from build123d import *

# Parameters (mm, degrees)
BOSS_EXTRUDE2_DEPTH = 3.175


with BuildPart() as part:
    # Sketch1 → Boss-Extrude2 (new body)
    # profile 1 of 7: a face of its own
    with BuildSketch(Plane(origin=(0, 0, 0), x_dir=(1, 0, 0), z_dir=(0, 1, 0))):
        with BuildLine():
            ThreePointArc((28.575, -5.499261314), (31.75, 0), (28.575, 5.499261314))
            ThreePointArc((28.575, 5.499261314), (5.55625, 9.6237073), (-9.525, 27.49630657))
            ThreePointArc((-9.525, 27.49630657), (-15.875, 27.49630657), (-19.05, 21.997045256))
            ThreePointArc((-19.05, 21.997045256), (-11.443597622, 4.764679711), (-14.037901317, -13.892259152))
            Line((-14.037901317, -13.892259152), (-12.274630657, -14.910283942))
            ThreePointArc((-12.274630657, -14.910283942), (-11.1125, -13.748153285), (-9.525, -13.322783942))
            Line((-9.525, -13.322783942), (-9.525, 13.322783942))
            ThreePointArc((-9.525, 13.322783942), (-11.77006403, 18.742847972), (-6.35, 16.497783942))
            ThreePointArc((-6.35, 16.497783942), (-6.458185502, 15.676033474), (-6.775369343, 14.910283942))
            Line((-6.775369343, 14.910283942), (16.300369343, 1.5875))
            ThreePointArc((16.300369343, 1.5875), (19.871750468, 3.066814498), (22.225, 0))
            ThreePointArc((22.225, 0), (19.871750468, -3.066814498), (16.300369343, -1.5875))
            Line((16.300369343, -1.5875), (-6.775369343, -14.910283942))
            ThreePointArc((-6.775369343, -14.910283942), (-6.458185502, -15.676033474), (-6.35, -16.497783942))
            ThreePointArc((-6.35, -16.497783942), (-6.458185502, -17.31953441), (-6.775369343, -18.085283942))
            Line((-6.775369343, -18.085283942), (-5.012098683, -19.103308732))
            ThreePointArc((-5.012098683, -19.103308732), (9.848132482, -7.528106395), (28.575, -5.499261314))
        make_face()
    # profile 2 of 7: a face of its own
    with BuildSketch(Plane(origin=(0, 0, 0), x_dir=(1, 0, 0), z_dir=(0, 1, 0))):
        with BuildLine():
            ThreePointArc((-9.525, -27.49630657), (-7.560164077, -23.143006881), (-5.012098683, -19.103308732))
            Line((-5.012098683, -19.103308732), (-6.775369343, -18.085283942))
            ThreePointArc((-6.775369343, -18.085283942), (-11.1125, -19.247414599), (-12.274630657, -14.910283942))
            Line((-12.274630657, -14.910283942), (-14.037901317, -13.892259152))
            ThreePointArc((-14.037901317, -13.892259152), (-16.262349841, -18.118797588), (-19.05, -21.997045256))
            ThreePointArc((-19.05, -21.997045256), (-15.875, -27.49630657), (-9.525, -27.49630657))
        make_face()
    # profile 3 of 7: a face of its own
    with BuildSketch(Plane(origin=(0, 0, 0), x_dir=(1, 0, 0), z_dir=(0, 1, 0))):
        with BuildLine():
            Line((-9.525, 13.322783942), (-9.525, -13.322783942))
            ThreePointArc((-9.525, -13.322783942), (-7.9375, -13.748153285), (-6.775369343, -14.910283942))
            Line((-6.775369343, -14.910283942), (16.300369343, -1.5875))
            ThreePointArc((16.300369343, -1.5875), (15.875, 0), (16.300369343, 1.5875))
            Line((16.300369343, 1.5875), (-6.775369343, 14.910283942))
            ThreePointArc((-6.775369343, 14.910283942), (-7.9375, 13.748153285), (-9.525, 13.322783942))
        make_face()
        with BuildLine():
            Line((-8.065819658, -1.523195628), (-8.065819658, 1.523195628))
            Line((-8.065819658, 1.523195628), (-6.298644043, 1.523195628))
            ThreePointArc((-6.298644043, 1.523195628), (-5.996260328, 2.457214638), (-5.55625, 3.334835474))
            Line((-5.55625, 3.334835474), (-5.55625, 8.0362073))
            ThreePointArc((-5.55625, 8.0362073), (-6.678782015, 10.746239315), (-3.96875, 9.6237073))
            ThreePointArc((-3.96875, 9.6237073), (-4.022842751, 9.212832065), (-4.181434671, 8.8299573))
            Line((-4.181434671, 8.8299573), (-0.109927238, 6.479271387))
            ThreePointArc((-0.109927238, 6.479271387), (3.240101916, 5.61202114), (5.666177238, 3.144435913))
            Line((5.666177238, 3.144435913), (9.737684671, 0.79375))
            ThreePointArc((9.737684671, 0.79375), (11.523375234, 1.533407249), (12.7, 0))
            ThreePointArc((12.7, 0), (11.523375234, -1.533407249), (9.737684671, -0.79375))
            Line((9.737684671, -0.79375), (5.666177238, -3.144435913))
            ThreePointArc((5.666177238, -3.144435913), (3.240101916, -5.61202114), (-0.109927238, -6.479271387))
            Line((-0.109927238, -6.479271387), (-4.181434671, -8.8299573))
            ThreePointArc((-4.181434671, -8.8299573), (-4.022842751, -9.212832065), (-3.96875, -9.6237073))
            ThreePointArc((-3.96875, -9.6237073), (-6.678782015, -10.746239315), (-5.55625, -8.0362073))
            Line((-5.55625, -8.0362073), (-5.55625, -3.334835474))
            ThreePointArc((-5.55625, -3.334835474), (-5.996260328, -2.457214638), (-6.298644043, -1.523195628))
            Line((-6.298644043, -1.523195628), (-8.065819658, -1.523195628))
        make_face(mode=Mode.SUBTRACT)
    # profile 4 of 7: a face of its own
    with BuildSketch(Plane(origin=(0, 0, 0), x_dir=(1, 0, 0), z_dir=(0, 1, 0))):
        with BuildLine():
            Line((-5.55625, 8.0362073), (-5.55625, 3.334835474))
            ThreePointArc((-5.55625, 3.334835474), (-3.240101916, 5.61202114), (-0.109927238, 6.479271387))
            Line((-0.109927238, 6.479271387), (-4.181434671, 8.8299573))
            ThreePointArc((-4.181434671, 8.8299573), (-4.7625, 8.248891971), (-5.55625, 8.0362073))
        make_face()
    # profile 5 of 7: a face of its own
    with BuildSketch(Plane(origin=(0, 0, 0), x_dir=(1, 0, 0), z_dir=(0, 1, 0))):
        with BuildLine():
            ThreePointArc((-0.109927238, -6.479271387), (-3.240101916, -5.61202114), (-5.55625, -3.334835474))
            Line((-5.55625, -3.334835474), (-5.55625, -8.0362073))
            ThreePointArc((-5.55625, -8.0362073), (-4.7625, -8.248891971), (-4.181434671, -8.8299573))
            Line((-4.181434671, -8.8299573), (-0.109927238, -6.479271387))
        make_face()
    # profile 6 of 7: a face of its own
    with BuildSketch(Plane(origin=(0, 0, 0), x_dir=(1, 0, 0), z_dir=(0, 1, 0))):
        with BuildLine():
            ThreePointArc((5.666177238, 3.144435913), (6.037080593, 2.355143226), (6.298644043, 1.523195628))
            Line((6.298644043, 1.523195628), (8.065819658, 1.523195628))
            Line((8.065819658, 1.523195628), (8.065819658, -1.523195628))
            Line((8.065819658, -1.523195628), (6.298644043, -1.523195628))
            ThreePointArc((6.298644043, -1.523195628), (6.037080593, -2.355143226), (5.666177238, -3.144435913))
            Line((5.666177238, -3.144435913), (9.737684671, -0.79375))
            ThreePointArc((9.737684671, -0.79375), (9.525, 0), (9.737684671, 0.79375))
            Line((9.737684671, 0.79375), (5.666177238, 3.144435913))
        make_face()
    # profile 7 of 7: a face of its own
    with BuildSketch(Plane(origin=(0, 0, 0), x_dir=(1, 0, 0), z_dir=(0, 1, 0))):
        with BuildLine():
            Line((-6.298644043, 1.523195628), (-8.065819658, 1.523195628))
            Line((-8.065819658, 1.523195628), (-8.065819658, -1.523195628))
            Line((-8.065819658, -1.523195628), (-6.298644043, -1.523195628))
            ThreePointArc((-6.298644043, -1.523195628), (-6.480203832, 0), (-6.298644043, 1.523195628))
        make_face()
    extrude(amount=BOSS_EXTRUDE2_DEPTH)


solid = part.part
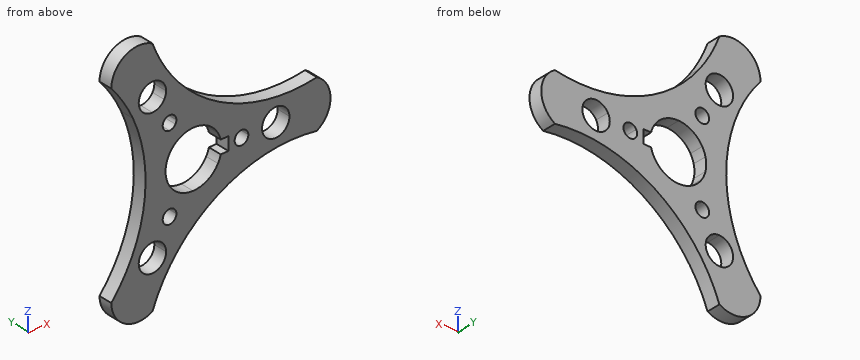
Could you check a few things on this model? Use its own coordinates, in mm. Give positions to 0.01 mm unless a question says otherwise; leave off trailing zeros. Order: outer loops, then holes, each group sorted by start corner. A loop starts at its lowest first (then second) coordinate and runs counter-clockwise, first axis right, second up. Notation, with made-up numbers: (-32.75, 10) - (-19.75, 10) arc R30 ccw to (-19.75, 45) - close; hole circle Ø8 at (-0.5, 1). An arc over 180 degrees is marked (long way). Return JSON: item names as keys, results as strings. Group by question number.
Q1. Will these pins go through, and if not, where does the flat tip stop? pin 1 Ø0.5 at (x, y) = (7.5, 2.5) entering from +Z; pin 2 Ø0.9 at (y, z) = (2, 0.5) entering from -X; pin 3 Ø1.4 at (x, y) = (7, 1.5) entering from -Z.
Q2. Suppose I cut it at B-B, the plane z = -10.5. Please give me the cut outline in (x, y) (3 decimals), and give its area (3 significant figures).
Q3. Suppose I cut it at C-C, the plane x = 2. Please give me the cut outline in (y, z) (3 decimals).
Q4. Please list where these lines run through material, in increasing order: line 1 along Z through (x, y) = (-9, 1.9); line 2 along Z through (x, y) = (-7, 0.55); line 3 along Z through (x, y) = (-6, 1.3). Write a range as [from, to].
Q5. Suppose I cut it at D-D, the plane y = 1.45. State how many separate pieces and enclosed holes the cut face has, and give its area (3 significant figures).
Q6. Suppose I cut it at A-A, the plane x = -10.5. Please give me the cut outline in (y, z) (3 decimals), and give its area (3 significant figures).
Resolved:
{
 "1": {"pin 1": "stops at z = 8.71", "pin 2": "stops at x = -11.13", "pin 3": "stops at z = -9.21"},
 "2": {"outline": "(-12.752, 0) - (-6.88, 0) - (-6.88, 3.175) - (-12.752, 3.175) - close; (-4.233, 0) - (4.121, 0) - (4.121, 3.175) - (-4.233, 3.175) - close", "area": "45.2 mm2"},
 "3": {"outline": "(0, -11.982) - (3.175, -11.982) - (3.175, -6.164) - (0, -6.164) - close; (0, 6.164) - (3.175, 6.164) - (3.175, 11.982) - (0, 11.982) - close"},
 "4": {"line 1": "z = [-26.16, -19.63], [-13.37, 13.37], [19.63, 26.16]", "line 2": "z = [-22.14, -18.42], [-14.57, -10.28], [-8.96, 8.96], [10.28, 14.57], [18.42, 22.14]", "line 3": "z = [-20.53, -11.15], [-8.1, -2.45], [2.45, 8.1], [11.15, 20.53]"},
 "5": {"separate pieces": "1", "enclosed holes": "7", "area": "831 mm2"},
 "6": {"outline": "(0, -27.954) - (3.175, -27.954) - (3.175, -19.519) - (0, -19.519) - close; (0, -13.476) - (3.175, -13.476) - (3.175, 13.476) - (0, 13.476) - close; (0, 19.519) - (3.175, 19.519) - (3.175, 27.954) - (0, 27.954) - close", "area": "139 mm2"}
}
